Verification items for this drawing (mm, ordinates from the low corner). Round coordinates to 2 decimals unless told otherwise and drop trailing zeros. Order: outer loops, then holes, each group sorted by start corner. A loop starts at its lowest first (then second) coordinate and runs counter-clockwise, first axis right, second up. Notation, with made-up numbers: M 86.5,-36 L 117.5,-36 A19 cw 117.5,0 Z; hole C 30.25,-30.5 d3. An arc over 180 degrees is marked long. Return JSON: item names as keys, results as strings. Group by question number.
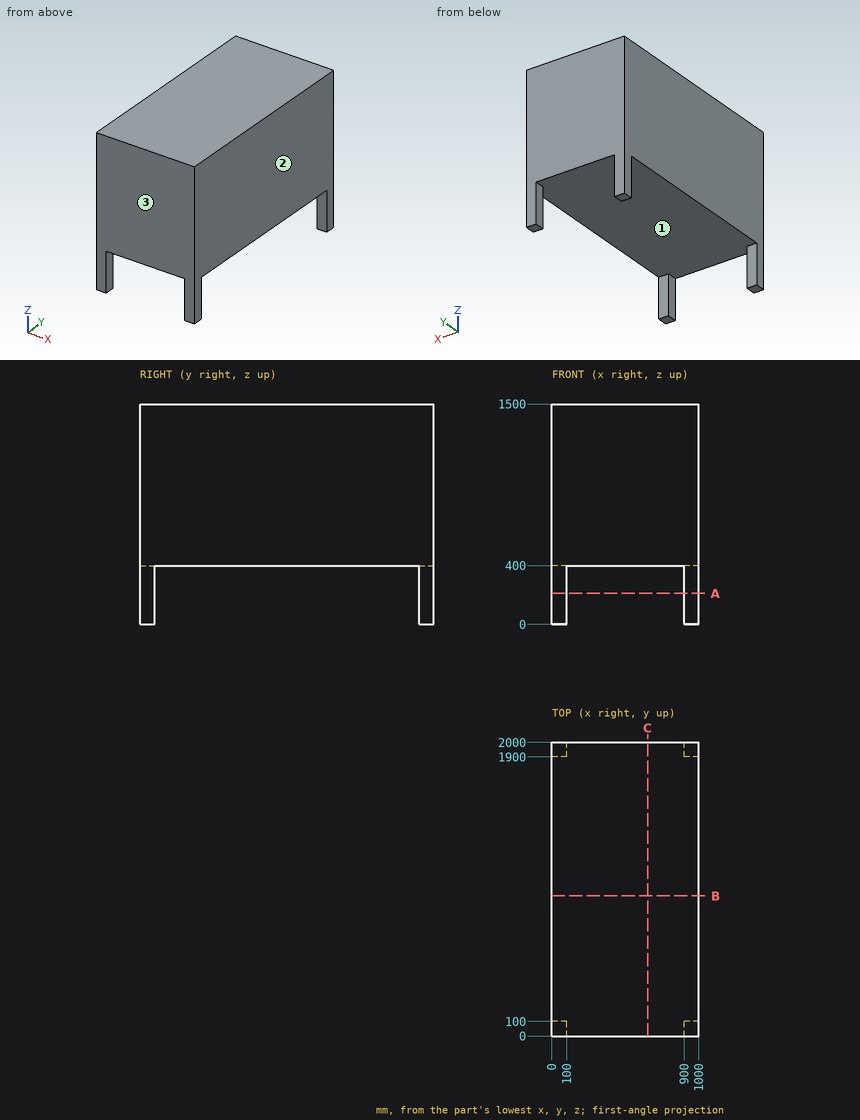
Q1. Depth check by flat-ended pin: pin 1 Ø6 at (x, y) = (307.5, 1323) entering from -Z. Enter the tip coordinate at first touch or a pass-through.
Q2. Section check C-C on x = 651.5. Record the cut outline in (y, z).
Q3. Section check B-B on y = 954. Record the cut outline in (x, z).
Q4. Material ranges on line 1 along Z through (x, y) = (203, 862), recorded low to high.
Q5. Release check for a two-part mould opening along Y. For the marked faces 1, 2 and 3 record: +Y half, -Y half, draft (parallel to the pull), parting line (faces both ways), or undercut.
Q6. Section check A-A on z = 211. Record the cut outline in (x, y).
Geometry check:
{
 "1": {"pin 1": "stops at z = 400"},
 "2": {"outline": "M 0,400 L 2000,400 L 2000,1500 L 0,1500 Z"},
 "3": {"outline": "M 0,400 L 1000,400 L 1000,1500 L 0,1500 Z"},
 "4": {"line 1": "z = 400 to 1500"},
 "5": {"face 1": "undercut", "face 2": "draft", "face 3": "-Y half"},
 "6": {"outline": "M 0,0 L 100,0 L 100,100 L 0,100 Z; M 0,1900 L 100,1900 L 100,2000 L 0,2000 Z; M 900,0 L 1000,0 L 1000,100 L 900,100 Z; M 900,1900 L 1000,1900 L 1000,2000 L 900,2000 Z"}
}
